```python
from build123d import *

# Parameters (mm, degrees)
F4_DEPTH = 25
F5_SIZE  = 0.5


with BuildPart() as f1:
    # F0 (on Front) → F1 (revolve)
    with BuildSketch(Plane.XZ):
        Polygon((-81.95, 3), (-81.95, 0), (-8.641222, 0), (-7.95, 1.3), (18.05, 1.3), (18.05, 1.95), (1.05, 1.95), (0, 3), align=None)
    revolve(axis=Axis((-31.95, 0, 0), (-1, 0, 0)))

    # F3 (on offset) → F4 (cut)
    with BuildSketch(Plane.XY.offset(3)):
        with BuildLine():
            ThreePointArc((-8.95, -0.39), (-11.07132, -5.51132), (-5.95, -3.39))
            Line((-5.95, -3.39), (-8.95, -3.39))
            Line((-8.95, -3.39), (-8.95, -0.39))
        make_face()
        with BuildLine():
            ThreePointArc((-8.95, -0.39), (-6.82868, -1.26868), (-5.95, -3.39))
            Line((-5.95, -3.39), (18.05, -3.39))
            Line((18.05, -3.39), (18.05, -1.95))
            Line((18.05, -1.95), (18.05, -0.39))
            Line((18.05, -0.39), (-8.95, -0.39))
        make_face()
        with BuildLine():
            Line((-8.95, -3.39), (-5.95, -3.39))
            ThreePointArc((-5.95, -3.39), (-6.82868, -1.26868), (-8.95, -0.39))
            Line((-8.95, -0.39), (-8.95, -3.39))
        make_face()
    extrude(amount=-F4_DEPTH, mode=Mode.SUBTRACT)

    # F5
    f5_edges = [f1.edges().sort_by_distance(p)[0] for p in [
        (-81.95, 0, -3),
    ]]
    chamfer(f5_edges, length=F5_SIZE)


solid = f1.part
```
Can you work these out from the model? Positions are in its coordinate system, mm. A direction names the side the tool comes from. Coordinates: 2 decimals unless noted, no trailing zeros. Loops run counter-clockwise (first coordinate to the right, second up) from the corner with the lowest first, then second, coordinate; pieces in that order, holes last. Notation, with made-up numbers: (50, -39.75) -> (66, -39.75) arc R28 ccw to (66, -1.75) -> close; hole circle Ø1 at (31, 35). An arc over 180 degrees is marked (long way). Answer as a JSON object with one key per item and string values.
1) Imagine slicing it at B-B (x = 4.5). Please give me the cut outline in (y, z), then the cut area to 3 significant figures.
Results:
{"outline": "(-0.39, -1.91) arc R1.95 ccw (long way) to (-0.39, 1.91) -> (-0.39, 1.24) arc R1.3 cw (long way) to (-0.39, -1.24) -> close", "area": "3.83 mm^2"}
2) Thinking about a two-plate mould opening in Y: for faces 1 (the face through (-41, 3, 0)), 2 (the face through (5.2, 1.3, 0)), 3 (the face through (-8.521, 0.224, -0.029)), 4 (the face through (-10.518, -0.833, 0.042)), which applies, pulls with the +Y half, pulls with the -Y half, needs draft (parallel to the pull), parting line crosses it, or undercut?
Results:
{"face 1": "parting line crosses it", "face 2": "undercut", "face 3": "undercut", "face 4": "pulls with the -Y half"}
3) For P1, Ø1, axis at x = -6.5, z = 2.5, coming from the +Y side; P2, Ø1, axis at x = -3.5, y = -1.5, coming from the -Z side; P3, Ø2.5, axis at y = 0, z = 0, coming from the +X side, each with a flat end and sliding along its axis, tell me the tip position at first contact or that it passes through.
Results:
{"P1": "stops at y = 2.24", "P2": "passes through", "P3": "stops at x = -7.98"}
4) Imagine slicing it at A-A (x = -35). Please give me the cut outline in (y, z).
Results:
{"outline": "circle Ø6 at (0, 0)"}
5) If I drill on line 1 (Z direction, x = 2.5, y = 0); line 2 (Z direction, x = -12.5, y = 0.25); line 3 (Y direction, x = 5, z = 0), over which ranges is the centre line in solid material (lowest first)?
Results:
{"line 1": "z = -1.95 to -1.3, 1.3 to 1.95", "line 2": "z = -2.99 to 2.99", "line 3": "y = 1.3 to 1.95"}
6) For faces 5 (the face through (18.05, 1.6, 0)), 6 (the face through (1.7, -0.39, 1.4)), which set-ups out of +Z, -Z, +X, -X, +Y, -Y let a thin tool reach every point of the face, with its end or its side?
Results:
{"face 5": "+Z, -Z, +X, +Y, -Y", "face 6": "+Z, -Z, +X, -Y"}
